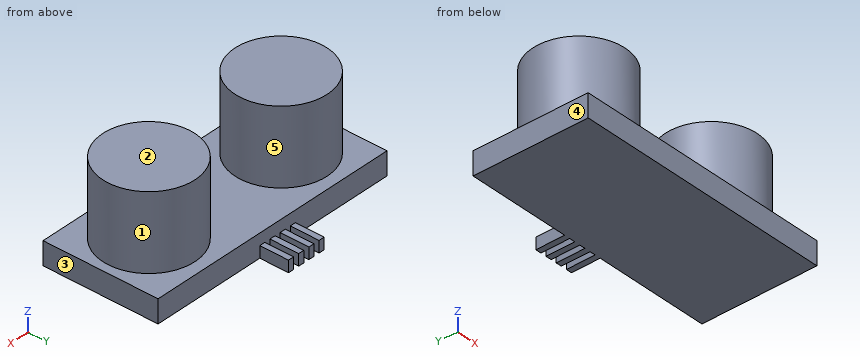
```python
from build123d import *

# Parameters (mm, degrees)
SKETCH1_W           = 45
SKETCH1_H           = 20
BOSS_EXTRUDE1_DEPTH = 4
SKETCH2_R           = 8
BOSS_EXTRUDE2_DEPTH = 13
BOSS_EXTRUDE3_DEPTH = 2


with BuildPart() as part:
    # Sketch1 → Boss-Extrude1 (new body)
    with BuildSketch(Plane.XY):
        Rectangle(SKETCH1_W, SKETCH1_H)
    extrude(amount=BOSS_EXTRUDE1_DEPTH)

    # Sketch2 → Boss-Extrude2 (add)
    with BuildSketch(Plane.XY.offset(4)):
        with Locations(Location((-13, 0, 0), (0, 0, 180))):
            Circle(SKETCH2_R)
        with Locations(Location((13, 0, 0), (0, 0, 180))):
            Circle(SKETCH2_R)
    extrude(amount=BOSS_EXTRUDE2_DEPTH)

    # Sketch4 → Boss-Extrude3 (add)
    with BuildSketch(Plane(origin=(0, 0, 0), x_dir=(-1, 0, 0), z_dir=(0, 0, -1))):
        Polygon((2, 15), (1.5, 15), (1.5, 10), (2.5, 10), (2.5, 15), align=None)
        Polygon((0, 15), (-0.5, 15), (-0.5, 10), (0.5, 10), (0.5, 15), align=None)
        Polygon((4, 15), (3.5, 15), (3.5, 10), (4.5, 10), (4.5, 15), align=None)
        Polygon((-2, 15), (-2.5, 15), (-2.5, 10), (-1.5, 10), (-1.5, 15), align=None)
    extrude(amount=-BOSS_EXTRUDE3_DEPTH)


solid = part.part
```
Geometry: final body of the model. Coordinates: model frame, mm. Face numbers are marked on the shaded views. A direction names the side the tool comes from. Give positions to 0.01 mm unless a question says otherwise; leave off trailing zeros. Loops run counter-clockwise (first coordinate to the right, second up) from the corner with the lowest first, then second, coordinate; pieces in that order, holes last. Notation, with made-up numbers: (50, 19) -> (109, 19) arc R31 cw to (109, 45) -> close; hole circle Ø5 at (-36.5, -9.75). An arc over 180 degrees is marked (long way). Use CSV: the item, a comma, the result in double quotes.
(1) First-contact query: P1, Ø1, axis at y = 12, z = 1, coming from the -X side; P2, Ø2, axis at x = -7, y = 10.5, coming from the -Z side; P3, Ø2, axis at x = 8, z = 1, coming from the +Y side; P4, Ø5, axis at y = 9.5, z = 10, coming from the -X side. Flat tips, straight axial feed; report the tip coordinate or a pass-through.
From the geometry:
P1,"x = -4.5"
P2,"z = 0"
P3,"y = 10"
P4,"x = -16.87"
(2) Access query for the marked faces 4 and 5. Directions: +Z, -Z, +X, -X, +Y, -Y. A direction counts if a zero-diameter tool reaches every point of the face in a straight line with its end or side. Return the directions, or none.
From the geometry:
face 4,"+Z, -Z, -X, +Y, -Y"
face 5,"+Z"
(3) Ray query, line 1 along Z through (x, y) = (14, 9.5); line 2 along Y through (x, z) = (-13, 12); line 3 along Y through (x, z) = (11, 2.5). Return the intervals inside material, ascending. Write a range as [from, to].
From the geometry:
line 1,"[0, 4]"
line 2,"[-8, 8]"
line 3,"[-10, 10]"
(4) Cut plane C-C (z = 14.5). Output: boundary loops of the cut face in (x, y).
From the geometry:
outline,"circle Ø16 at (-13, 0); circle Ø16 at (13, 0)"
(5) Pull-direction query (X, two-part tool) for the marked faces 1, 2 and 3; classes: released by +X, released by -X, zero draft, split by the parting line, or undercut.
From the geometry:
face 1,"undercut"
face 2,"zero draft"
face 3,"released by +X"
(6) Cut plane B-B (x = 2). Output: boundary loops of the cut face in (y, z), plus the area to 3 significant figures.
From the geometry:
outline,"(-10, 0) -> (15, 0) -> (15, 2) -> (10, 2) -> (10, 4) -> (-10, 4) -> close"
area,"90.0 mm^2"
(7) Cut plane A-A (y = 0). Output: boundary loops of the cut face in (x, z), plus the area to 3 significant figures.
From the geometry:
outline,"(-22.5, 0) -> (22.5, 0) -> (22.5, 4) -> (21, 4) -> (21, 17) -> (5, 17) -> (5, 4) -> (-5, 4) -> (-5, 17) -> (-21, 17) -> (-21, 4) -> (-22.5, 4) -> close"
area,"596 mm^2"
(8) Cut plane D-D (x = 16.5). Output: boundary loops of the cut face in (y, z), plus the area to 3 significant figures.
From the geometry:
outline,"(-10, 0) -> (10, 0) -> (10, 4) -> (7.19, 4) -> (7.19, 17) -> (-7.19, 17) -> (-7.19, 4) -> (-10, 4) -> close"
area,"267 mm^2"
